Input: part model. Units: mm. Frame: model coordinates. Face numbers are marked on the shaded views. Round coordinates to 2 decimals unless told otherwise and drop trailing zeros. Order: outer loops, then holes, each group sorted by start corner. A loop starts at its lowest first (then second) coordinate and runs counter-clockwise, first axis right, second up. Notation, with made-up numbers: M -38,-31 L -31,-31 A7 ccw -31,-20 Z; hole C 54,-35.75 d7. An arc over 180 degrees is marked long. One line per question, with ' | ' between items.
```python
from build123d import *

# Parameters (mm, degrees)
SKETCH1_W            = 82
SKETCH1_H            = 58
SKETCH1_R            = 12.6
SKETCH1_R_2          = 6.1
BOSS_EXTRUDE1_DEPTH  = 8
FILLET1_R            = 10
FILLET1_OF_MIRROR1_R = 10
SKETCH2_W            = 82
SKETCH2_H            = 58
CUT_EXTRUDE1_DEPTH   = 175.137876408


with BuildPart() as part:
    # Sketch1 → Boss-Extrude1 (new body)
    with BuildSketch(Plane(origin=(0, 0, 0), x_dir=(1, 0, 0), z_dir=(0, 1, 0))):
        with Locations((41, 29)):
            Rectangle(SKETCH1_W, SKETCH1_H)
        with Locations(Location((23.5, 29, 0), (0, 0, 270))):
            Circle(SKETCH1_R, mode=Mode.SUBTRACT)
        with Locations(Location((68.57, 48, 0), (0, 0, 270))):
            Circle(SKETCH1_R_2, mode=Mode.SUBTRACT)
        with Locations(Location((54.561074274, 10, 0), (0, 0, 270))):
            Circle(SKETCH1_R_2, mode=Mode.SUBTRACT)
        with Locations(Location((12.561074274, 10, 0), (0, 0, 270))):
            Circle(SKETCH1_R_2, mode=Mode.SUBTRACT)
        with Locations(Location((12.561074274, 48, 0), (0, 0, 270))):
            Circle(SKETCH1_R_2, mode=Mode.SUBTRACT)
    boss_extrude1 = extrude(amount=BOSS_EXTRUDE1_DEPTH)

    # Fillet1
    fillet1_edges = [part.edges().sort_by_distance(p)[0] for p in [
        (0, 4, 0),
        (0, 4, -58),
        (82, 4, -58),
        (82, 4, 0),
    ]]
    fillet(fillet1_edges, radius=FILLET1_R)


with BuildPart() as mirror1_1:
    # Mirror1: Boss-Extrude1 across plane
    add(boss_extrude1.mirror(Plane(origin=(82, 8, 0), x_dir=(0, 0, 1), z_dir=(-1, 0, 0))))

    # Fillet1 of Mirror1
    fillet1_of_mirror1_edges = [mirror1_1.edges().sort_by_distance(p)[0] for p in [
        (164, 4, 0),
        (164, 4, -58),
        (82, 4, -58),
        (82, 4, 0),
    ]]
    fillet(fillet1_of_mirror1_edges, radius=FILLET1_OF_MIRROR1_R)


with BuildPart() as part_1:
    add(part.part)

    # Mirror1 united with what the copies touc: union Mirror1_1
    add(mirror1_1.part)

    # Sketch2 → Cut-Extrude1 (cut, through all)
    with BuildSketch(Plane(origin=(0, 8, 0), x_dir=(1, 0, 0), z_dir=(0, 1, 0))):
        with Locations((41, 29)):
            Rectangle(SKETCH2_W, SKETCH2_H)
    extrude(amount=-CUT_EXTRUDE1_DEPTH, mode=Mode.SUBTRACT)


solid = part_1.part
```
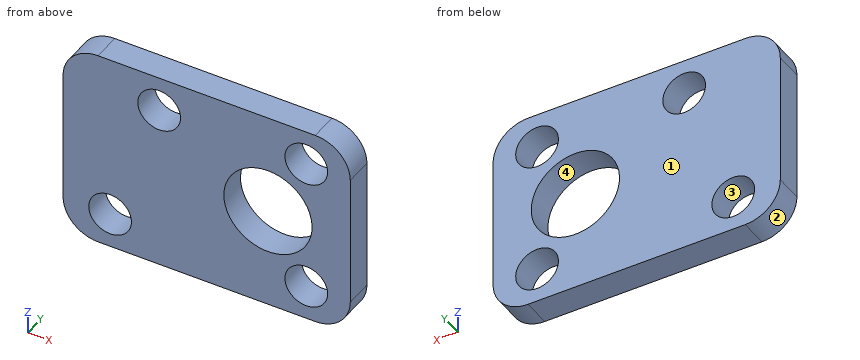
Item 1: Section query A-A, the plane x = 140.5. Return loops of the section in (y, z), plus the area to 3 significant figures.
Report:
outline: M 0,-58 L 8,-58 L 8,-41.6 L 0,-41.6 Z; M 0,-16.4 L 8,-16.4 L 8,0 L 0,0 Z | area: 262 mm²
Item 2: Section query D-D, the plane y = 7. Return loops of the section in (x, z).
Report:
outline: M 82,-48 A10 ccw 92,-58 L 154,-58 A10 ccw 164,-48 L 164,-10 A10 ccw 154,0 L 92,0 A10 ccw 82,-10 Z; hole C 95.43,-48 d12.2; hole C 109.44,-10 d12.2; hole C 140.5,-29 d25.2; hole C 151.44,-48 d12.2; hole C 151.44,-10 d12.2
Item 3: Line query: line 1 along X through (y, z) = (5.5, -48); line 2 along Z through (x, y) = (140.5, 5.75); line 3 along Z through (x, y) = (109, 2). Output: solid intervals per line, ascending. Write a range as from..to.
Report:
line 1: 82..89.33, 101.53..145.34, 157.54..164 | line 2: -58..-41.6, -16.4..0 | line 3: -58..-16.08, -3.92..0
Item 4: Section query C-C, the plane z = -7. Return loops of the section in (x, y), plus the area to 3 significant figures.
Report:
outline: M 82.46,0 L 104.13,0 L 104.13,8 L 82.46,8 Z; M 114.75,0 L 146.13,0 L 146.13,8 L 114.75,8 Z; M 156.75,0 L 163.54,0 L 163.54,8 L 156.75,8 Z | area: 479 mm²
Item 5: Section query B-B, the plane z = -29. Return loops of the section in (x, y).
Report:
outline: M 82,0 L 127.9,0 L 127.9,8 L 82,8 Z; M 153.1,0 L 164,0 L 164,8 L 153.1,8 Z
Item 6: Mould query, pull axis Z, two halves, no side actions, for the marked faces 1, 2, 3 and 4. Classes: +Z half, -Z half, draft (parallel to the pull), parting line (faces both ways), or undercut.
Report:
face 1: draft | face 2: -Z half | face 3: undercut | face 4: undercut
